Can you work these out from the drawing? Everything is in mm from the part's minimum corner. A direction names the side the tool comes from. Coordinates: 2 decimals unless noted, no trailing zeros. Loops run counter-clockwise (first coordinate to the right, second up) from the corner with the lowest first, then second, coordinate; pieces in that order, holes last. Notation, with made-up numbers: (-29.75, 61) -> (27.25, 61) arc R14 ccw to (27.25, 80) -> close; hole circle Ø5 at (54.5, -12.5). An arc over 180 degrees is marked (long way). Put each result on its own line as item: value. Start each with the question number.
Item 1: If we section it at C-C on y = 2.5: Please give me the cut outline in (x, z).
Item 2: If we section it at D-D on z = 3: Please give me the cut outline in (x, y), plus the area to 3 significant figures.
Item 3: If we section it at B-B on x = 3.5: Please give me the cut outline in (y, z).
Item 4: Please list where these lines run through material, in increasing order: L1, parallel to Y at x = 3.5, z = 1.9; L2, parallel to Y at x = 3.5, z = 3.8; L3, parallel to X at y = 2.5, z = 3.25. Write a range as from..to.
Item 5: We'd pull the mould along Y, two halves only. Please class the marked faces 3, 4 and 5: pulls with the +Y half, pulls with the -Y half, needs draft (parallel to the pull), parting line crosses it, or undercut.
Item 6: For the marked faces 1 and 2, which set-ups out of +Z, -Z, +X, -X, +Y, -Y let a thin tool reach every point of the face, with its end or its side?
Item 7: Will this pin go through, and if not, where does the flat tip stop? P1, Ø3.5, axis at x = 3.5, y = 2.5, coming from the +Z side.
Item 8: If we section it at A-A on y = 37.5: Please give me the cut outline in (x, z), plus the area to 3 significant figures.
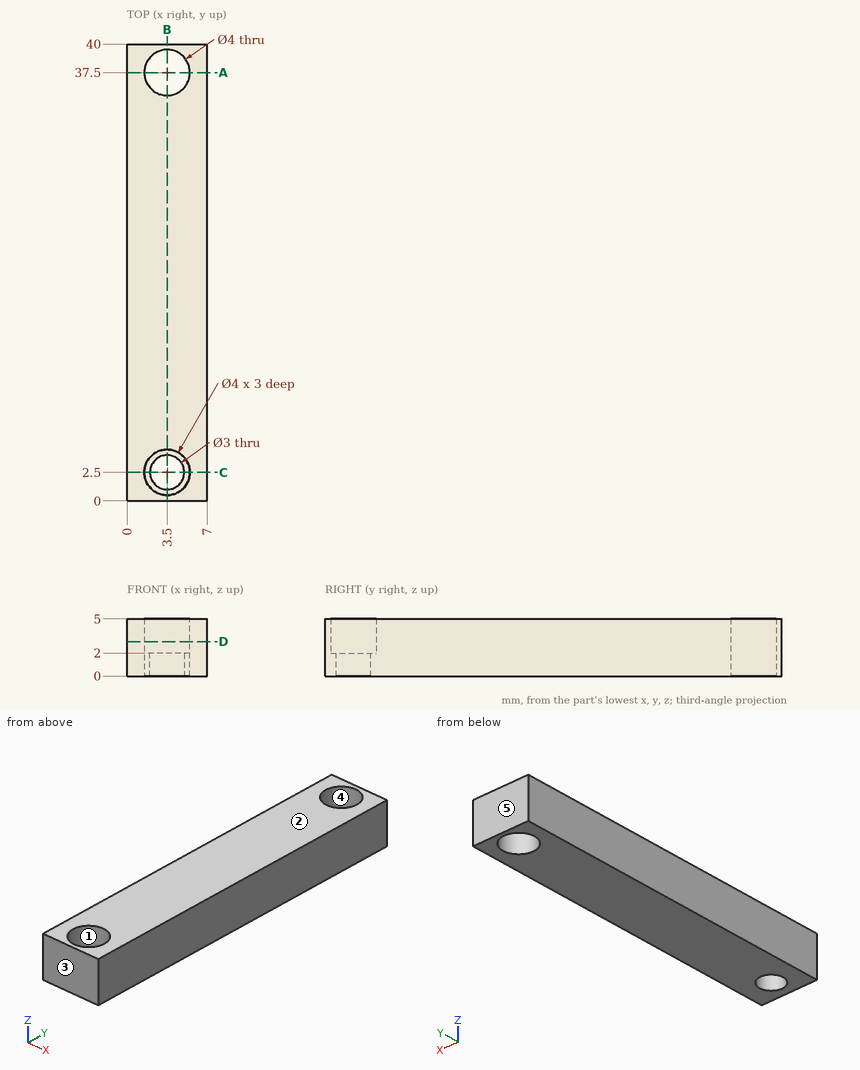
Solutions:
1. outline: (0, 0) -> (2, 0) -> (2, 2) -> (1.5, 2) -> (1.5, 5) -> (0, 5) -> close; (5, 0) -> (7, 0) -> (7, 5) -> (5.5, 5) -> (5.5, 2) -> (5, 2) -> close
2. outline: (0, 0) -> (7, 0) -> (7, 40) -> (0, 40) -> close; hole circle Ø4 at (3.5, 2.5); hole circle Ø4 at (3.5, 37.5)
2. area: 255 mm^2
3. outline: (0, 0) -> (1, 0) -> (1, 2) -> (0.5, 2) -> (0.5, 5) -> (0, 5) -> close; (4, 0) -> (35.5, 0) -> (35.5, 5) -> (4.5, 5) -> (4.5, 2) -> (4, 2) -> close; (39.5, 0) -> (40, 0) -> (40, 5) -> (39.5, 5) -> close
4. L1: 0..1, 4..35.5, 39.5..40
4. L2: 0..0.5, 4.5..35.5, 39.5..40
4. L3: 0..1.5, 5.5..7
5. face 3: pulls with the -Y half
5. face 4: undercut
5. face 5: pulls with the +Y half
6. face 1: +Z
6. face 2: +Z, +X, -X, +Y, -Y
7. P1: z = 2
8. outline: (0, 0) -> (1.5, 0) -> (1.5, 5) -> (0, 5) -> close; (5.5, 0) -> (7, 0) -> (7, 5) -> (5.5, 5) -> close
8. area: 15.0 mm^2
